Verification items for the finished model (mm, model axes). Give positions to 0.01 mm unless a question says otherwise; leave off trailing zeros. Loops run counter-clockwise (first coordinate to the right, second up) from the corner with the lowest first, then second, coordinate; pieces in that order, holes last. Notation, with made-up numbers: M 18.5,28.25 L 38.5,28.25 A19 ccw 38.5,35.25 Z; hole C 72,-8 d4. An arc over 180 degrees is marked long. Use a Markdown table: item, result.
from build123d import *

# Parameters (mm, degrees)
SKETCH1_W           = 740
SKETCH1_H           = 608
SKETCH1_R           = 12.5
SKETCH1_R_2         = 1.5
SKETCH1_W_2         = 610
SKETCH1_H_2         = 535
BOSS_EXTRUDE1_DEPTH = 5


with BuildPart() as part:
    # Sketch1 → Boss-Extrude1 (new body)
    with BuildSketch(Plane(origin=(0, 0, 0), x_dir=(1, 0, 0), z_dir=(0, 1, 0))):
        with Locations((370, 304)):
            Rectangle(SKETCH1_W, SKETCH1_H)
        with Locations(Location((40, 559, 0), (0, 0, 270))):
            Circle(SKETCH1_R, mode=Mode.SUBTRACT)
        with Locations(Location((40, 49, 0), (0, 0, 270))):
            Circle(SKETCH1_R, mode=Mode.SUBTRACT)
        with Locations(Location((25, 64, 0), (0, 0, 270))):
            Circle(SKETCH1_R_2, mode=Mode.SUBTRACT)
        with Locations(Location((25, 34, 0), (0, 0, 270))):
            Circle(SKETCH1_R_2, mode=Mode.SUBTRACT)
        with Locations(Location((55, 34, 0), (0, 0, 270))):
            Circle(SKETCH1_R_2, mode=Mode.SUBTRACT)
        with Locations(Location((55, 64, 0), (0, 0, 270))):
            Circle(SKETCH1_R_2, mode=Mode.SUBTRACT)
        with Locations(Location((25, 574, 0), (0, 0, 270))):
            Circle(SKETCH1_R_2, mode=Mode.SUBTRACT)
        with Locations(Location((55, 574, 0), (0, 0, 270))):
            Circle(SKETCH1_R_2, mode=Mode.SUBTRACT)
        with Locations(Location((55, 544, 0), (0, 0, 270))):
            Circle(SKETCH1_R_2, mode=Mode.SUBTRACT)
        with Locations(Location((25, 544, 0), (0, 0, 270))):
            Circle(SKETCH1_R_2, mode=Mode.SUBTRACT)
        with Locations((385, 304)):
            Rectangle(SKETCH1_W_2, SKETCH1_H_2, mode=Mode.SUBTRACT)
    extrude(amount=BOSS_EXTRUDE1_DEPTH)


solid = part.part
(1) Cross-section at B-B on x = 354. Record the cut outline in (y, z), then the cut area to 3 significant figures.
Results below:
| item | result |
|---|---|
| outline | M 0,-608 L 5,-608 L 5,-571.5 L 0,-571.5 Z; M 0,-36.5 L 5,-36.5 L 5,0 L 0,0 Z |
| area | 365 mm^2 |
(2) Draft check along Z on faces 1 (the cylindrical face through (32.394, 2.465, -58.92)), 2 (the flat face through (341, 5, -35)). Enter one of: +Z half, -Z half, draft (parallel to the pull), parting line (faces both ways), or undercut.
Results below:
| item | result |
|---|---|
| face 1 | undercut |
| face 2 | draft |
(3) Material ranges on line 1 (X direction, y = 4, z = -544); line 2 (Z direction, x = 302, y = 0.3); line 3 (X direction, y = 3.25, z = -473), recorded low to high.
Results below:
| item | result |
|---|---|
| line 1 | 0 to 23.5, 26.5 to 53.5, 56.5 to 80, 690 to 740 |
| line 2 | -608 to -571.5, -36.5 to 0 |
| line 3 | 0 to 80, 690 to 740 |
(4) Cross-section at C-C on z = -49. Record the cut outline in (x, y).
Results below:
| item | result |
|---|---|
| outline | M 0,0 L 27.5,0 L 27.5,5 L 0,5 Z; M 52.5,0 L 80,0 L 80,5 L 52.5,5 Z; M 690,0 L 740,0 L 740,5 L 690,5 Z |
(5) Gauge pin test, flat end, axial feed: P1, Ø1.8, axis at x = 25, z = -34, coming from the +Y side. Record the tip position at first contact, or that the pin passes through.
Results below:
| item | result |
|---|---|
| P1 | through |
(6) Cross-section at A-A on x = 40. Record the cut outline in (y, z), then the cut area to 3 significant figures.
Results below:
| item | result |
|---|---|
| outline | M 0,-608 L 5,-608 L 5,-571.5 L 0,-571.5 Z; M 0,-546.5 L 5,-546.5 L 5,-61.5 L 0,-61.5 Z; M 0,-36.5 L 5,-36.5 L 5,0 L 0,0 Z |
| area | 2,790 mm^2 |
(7) Cross-section at D-D on y = 2.5. State how many separate pieces and enclosed holes the cut face has, then the cut area to 3 significant figures.
Results below:
| item | result |
|---|---|
| separate pieces | 1 |
| enclosed holes | 11 |
| area | 123,000 mm^2 |
